Build history of the part. All positions in model axes, mm. Face numbers are marked on the shaded views. A direction names the side the tool comes from. Give positions to 0.01 mm unless a question says otherwise; leave off trailing zeros. Loops run counter-clockwise (first coordinate to the right, second up) from the corner with the lowest first, then second, coordinate; pieces in that order, holes last. Notation, with made-up numbers: (-11.5, 4) -> (41.5, 4) arc R15 ccw to (41.5, 12) -> close; hole circle Ø7 at (43, 67). An arc over 180 degrees is marked (long way). Answer as a JSON object with one key per item and string values. Group by question number.
Q1. Band-saw the part on B-B, the plane z = 0. Write the cut outline in (x, y).
Q2. Drop flat-ended pins along their axis: pin 1 (1 mm diameter, centred on x = -8, z = -0.5, fed in from +Y); pin 2 (1.5 mm diameter, centred on y = 92.5, z = 162.5, fed in from +X); pin 3 (3 mm diameter, centred on x = -147.5, y = 106, fed in from -Z). Give the stop position or say it passes through.
Q3. Band-saw the part on D-D, the plane z = -69. Count the separate pieces of the cut face and the enclosed holes in it, plus the area to 3 significant figures.
Q4. Wall check: probe 1 along Z at (x, y) = (0, 107); probe 2 along Y at (x, z) = (-206, -115). Give the ranges that are in metal, low to high. Write a range as from..to.
Q5. Band-saw the part on C-C, the plane y = 84.5. Write the cut outline in (x, z).
Q6. Band-saw the part on A-A, the plane x = 0. Write the cut outline in (y, z).
Q7. Tool access for the marked faces 4 and 5: list every direction of +Z, -Z, +X, -X, +Y, -Y with a clear straight run to the whole face (end or side of a thin tool).
Q8. Two-plate mould, pull along Z, no slides. Class the marked faces 1, 2 and 3: pulls with the +Z half, pulls with the -Z half, needs draft (parallel to the pull), parting line crosses it, or undercut.
Autodesk Inventor part; units mm, degrees
ref_plane "YZ Plane" through (0, 0, 0) normal (1, 0, 0) x (0, 1, 0)
ref_plane "XZ Plane" through (0, 0, 0) normal (0, 1, 0) x (-1, 0, 0)
ref_plane "XY Plane" through (0, 0, 0) normal (0, 0, 1) x (1, 0, 0)
sketch "Sketch1" plane through (0, 0, 0) normal (0, 0, 1) x (1, 0, 0)
  line L0 (320, 126) -> (320, 70)
  line L1 (320, 70) -> (285.9746, 21.3454)
  arc A0 (245, 0) -> (285.9746, 21.3454) centre (245, 50) ccw
  line L2 (245, 0) -> (0, 0)
  line L3 (320, 129) -> (320, 126)
  line L4 (0, -2) -> (245, -2)
  arc A1 (245, -2) -> (287.6135, 20.1992) centre (245, 50) ccw
  line L5 (287.6135, 20.1992) -> (322, 69.3701)
  line L6 (322, 69.3701) -> (322, 126)
  line L7 (322, 126) -> (322, 129)
  line L8 (322, 129) -> (320, 129)
  line L9 (0, -25.8) -> (0, 154.8) construction
  line L10 (0, 0) -> (0, -2)
  point P0 (0, 0)
  dimension "d0" = 2
  dimension "d1" = 30.4542
revolve "Revolution1" add sketch "Sketch1" angle 360 about axis through (0, -25.8, 0) along (0, 1, 0)
sketch "Sketch2" plane through (0, 0, 0) normal (0, 1, 0) x (1, 0, 0)
  circle A0 centre (0, -138) radius 12
  circle A1 centre (119.5115, 69) radius 12
  circle A2 centre (-119.5115, 69) radius 12
  point P0 (0, 0)
extrude "Extrusion1" cut sketch "Sketch2" against normal through all
properties part number "coating"
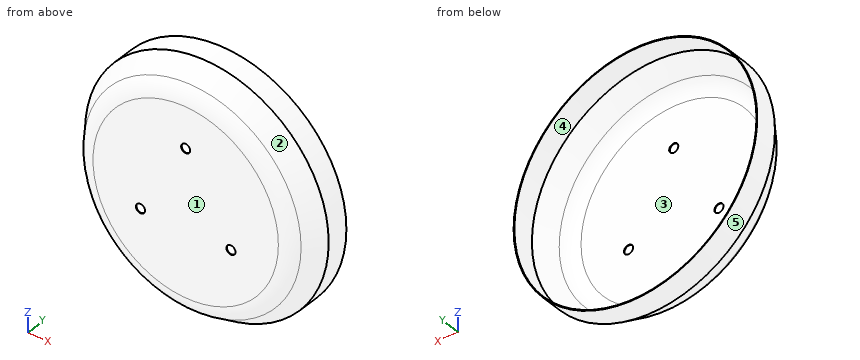
Worked answers:
{
 "1": {"outline": "(-322, 69.37) -> (-287.61, 20.2) arc R52 ccw to (-245, -2) -> (245, -2) arc R52 ccw to (287.61, 20.2) -> (322, 69.37) -> (322, 129) -> (320, 129) -> (320, 70) -> (285.97, 21.35) arc R50 cw to (245, 0) -> (-245, 0) arc R50 cw to (-285.97, 21.35) -> (-320, 70) -> (-320, 129) -> (-322, 129) -> close"},
 "2": {"pin 1": "y = 0", "pin 2": "x = 278.43", "pin 3": "z = -287"},
 "3": {"separate pieces": "3", "enclosed holes": "0", "area": "1,540 mm2"},
 "4": {"probe 1": "-322..-320, 320..322", "probe 2": "-2..0"},
 "5": {"outline": "circle Ø644 at (0, 0); hole circle Ø640 at (0, 0)"},
 "6": {"outline": "(-2, -245) arc R52 ccw to (20.2, -287.61) -> (69.37, -322) -> (129, -322) -> (129, -320) -> (70, -320) -> (21.35, -285.97) arc R50 cw to (0, -245) -> (0, 126) -> (-2, 126) -> close; (-2, 150) -> (0, 150) -> (0, 245) arc R50 cw to (21.35, 285.97) -> (70, 320) -> (129, 320) -> (129, 322) -> (69.37, 322) -> (20.2, 287.61) arc R52 ccw to (-2, 245) -> close"},
 "7": {"face 4": "+Y", "face 5": "+Y, -Y"},
 "8": {"face 1": "needs draft", "face 2": "parting line crosses it", "face 3": "undercut"}
}
